Verification items for the finished model (mm, model axes). A direction names the side the tool comes from. Coordinates: 2 decimals unless noted, no trailing zeros. Order: outer loops, then holes, each group sorted by start corner. A loop starts at its lowest first (then second) coordinate and runs counter-clockwise, first axis right, second up. Notation, with made-up numbers: (-14.75, 48) - (25.25, 48) arc R22 ccw to (25.25, 87) - close; hole circle Ø9 at (74.25, 34). An arc over 180 degrees is marked (long way). One line per question, with ' | ' between items. Start each with the question number.
Autodesk Inventor part; units mm, degrees
ref_plane "C3_XY" through (131, 0, 0) normal (-1, 0, 0) x (0, 0, -1)
ref_plane "C3_YZ" through (131, 0, 0) normal (0, 0, -1) x (0, -1, 0)
ref_plane "C3_ZX" through (131, 0, 0) normal (0, -1, 0) x (-1, 0, 0)
sketch "Sketch_1" plane through (0, 0, 0) normal (0, 0, 1) x (1, 0, 0)
  line L0 (131, 0) -> (0, 0)
  line L1 (0, 0) -> (0, 3.5)
  line L2 (0, 3.5) -> (0.6062, 4.55)
  line L3 (0.6062, 4.55) -> (130.3938, 4.55)
  line L4 (130.3938, 4.55) -> (131, 3.5)
  line L5 (131, 3.5) -> (131, 0)
  line L6 (131, 0) -> (0, 0)
revolve "Revolution1" add sketch "Sketch_1" angle 360 about axis through (131, 0, 0) along (1, 0, 0)
sketch "Sketch_2" plane through (0, 0, 0) normal (1, 0, 0) x (0, 1, 0)
  line L0 (7, 7) -> (-7, 7)
  line L1 (-7, 7) -> (-7, -7)
  line L2 (-7, -7) -> (7, -7)
  line L3 (7, -7) -> (7, 7)
  line L4 (-2.0207, 3.5) -> (-4.0415, 0)
  line L5 (-4.0415, 0) -> (-2.0207, -3.5)
  line L6 (-2.0207, -3.5) -> (2.0207, -3.5)
  line L7 (2.0207, -3.5) -> (4.0415, 0)
  line L8 (4.0415, 0) -> (2.0207, 3.5)
  line L9 (2.0207, 3.5) -> (-2.0207, 3.5)
extrude "Extrusion1" cut sketch "Sketch_2" along normal blind 131
sketch "Sketch3" plane through (0, 0, 0) normal (-1, 0, 0) x (0, 0, 1)
  point P0 (0, 0)
hole "Hole1" at (0, 0, 0) direction (1, 0, 0) diameter 2.459 depth 8.2901 tip angle 120 countersink diameter 3 countersink angle 90
sketch "Sketch4" plane through (131, 0, 0) normal (1, 0, 0) x (0, 0, -1)
  point P0 (0, 0)
hole "Hole2" at (131, 0, 0) direction (-1, 0, 0) diameter 2.459 depth 8.2901 tip angle 120 countersink diameter 3 countersink angle 90
ref_plane "C3_XY" through (131, 0, 0) normal (-1, 0, 0) x (0, 0, -1)
ref_plane "C3_YZ" through (131, 0, 0) normal (0, 0, -1) x (0, -1, 0)
ref_plane "C3_ZX" through (131, 0, 0) normal (0, -1, 0) x (-1, 0, 0)
properties part number "SLSBF7-131-M3-N3"
Item 1: Section check A-A (x = 85). Record the cut outline in (y, z), then the cut area to 3 significant figures.
Item 2: Set-up check for faces 1 (the flat face through (65, 0, -3.5)), 2 (the cylindrical face through (4.336, 0.748, -0.976)), 3 (the cylindrical face through (126.664, 0.748, 0.976)): record each of +Z, -Z, +X, -X, +Y, -Y from which the full face is reachable in a straight line by a thin tool's end or side.
Item 3: Gauge pin test, flat end, axial feed: pin 1 (1.5 mm diameter, centred on x = 79.5, z = 2.5, fed in from +Y). Record the tip position at first contact, or that the pin passes through.
Item 4: Thickness scan on probe 1 along Z at (x, y) = (126.25, 0); probe 2 along Y at (x, z) = (127.5, 0); probe 3 along Z at (x, y) = (5.5, 1). Record the ranges inside material, lowest first. Write a range as from..to.
Item 5: Mould release check, pull along Y, two halves, no side actions. Record for faces 4 (the conical face through (9, 0, 0)), 5 (the flat face through (65, 0, 3.5)), 6 (the flat face through (64.6, -3, 1.8)): +Y half, -Y half, draft (parallel to the pull), parting line (faces both ways), or undercut.
Completed:
1) outline: (-4.04, 0) - (-2.02, -3.5) - (2.02, -3.5) - (4.04, 0) - (2.02, 3.5) - (-2.02, 3.5) - close | area: 42.4 mm^2
2) face 1: -Z, +X, -X, +Y, -Y | face 2: -X | face 3: +X
3) pin 1: stops at y = 3.03
4) probe 1: z = -3.5..-1.23, 1.23..3.5 | probe 2: y = -4.04..-1.23, 1.23..4.04 | probe 3: z = -3.5..-0.72, 0.72..3.5
5) face 4: undercut | face 5: draft | face 6: -Y half
